```python
from build123d import *

# Parameters (mm, degrees)
F1_DEPTH = 3.175
F2_W     = 62.6118863001
F2_H     = 3.175
F3_DEPTH = 12.7
F4_SIZE  = 1.27
F5_W     = 15.875
F5_H     = 3.175
F6_DEPTH = 4.5143370517
F7_W     = 15.875
F7_H     = 3.175
F8_DEPTH = 4.3210691154


with BuildPart() as f1:
    # F0 (on Front) → F1 (new body)
    with BuildSketch(Plane.XZ):
        with BuildLine():
            ThreePointArc((-35.500738686, -3.175), (-34.8663710031, -1.6435009364), (-34.65, 0))
            Line((-34.65, 0), (-39.5, 0))
            ThreePointArc((-39.5, 0), (-41, -1.5), (-42.5, 0))
            Line((-42.5, 0), (-47.35, 0))
            ThreePointArc((-47.35, 0), (-47.1336289969, -1.6435009364), (-46.499261314, -3.175))
            Line((-46.499261314, -3.175), (-35.500738686, -3.175))
        make_face()
        with BuildLine():
            ThreePointArc((-40.777693324, 6.346107448), (-36.4319507778, 4.4108305685), (-34.65, 0))
            Line((-34.65, 0), (-6.35, 0))
            ThreePointArc((-6.35, 0), (-4.5680492222, 4.4108305685), (-0.222306676, 6.346107448))
            Line((-0.222306676, 6.346107448), (-40.777693324, 6.346107448))
        make_face()
        with BuildLine():
            Line((-39.5, 0), (-34.65, 0))
            ThreePointArc((-34.65, 0), (-36.4319507778, 4.4108305685), (-40.777693324, 6.346107448))
            ThreePointArc((-40.777693324, 6.346107448), (-45.4108305685, 4.5680492222), (-47.35, 0))
            Line((-47.35, 0), (-42.5, 0))
            ThreePointArc((-42.5, 0), (-41, 1.5), (-39.5, 0))
        make_face()
        with BuildLine():
            ThreePointArc((-46.499261314, -3.175), (-47.1336289969, -1.6435009364), (-47.35, 0))
            Line((-47.35, 0), (-47.35, -3.175))
            Line((-47.35, -3.175), (-46.499261314, -3.175))
        make_face()
        with BuildLine():
            ThreePointArc((-0.222306676, 6.346107448), (-4.5680492222, 4.4108305685), (-6.35, 0))
            Line((-6.35, 0), (-1.5, 0))
            ThreePointArc((-1.5, 0), (0, 1.5), (1.5, 0))
            Line((1.5, 0), (6.35, 0))
            ThreePointArc((6.35, 0), (4.4108305685, 4.5680492222), (-0.222306676, 6.346107448))
        make_face()
        with BuildLine():
            Line((-1.5, 0), (-6.35, 0))
            ThreePointArc((-6.35, 0), (-6.1336289969, -1.6435009364), (-5.499261314, -3.175))
            Line((-5.499261314, -3.175), (5.499261314, -3.175))
            ThreePointArc((5.499261314, -3.175), (6.1336289969, -1.6435009364), (6.35, 0))
            Line((6.35, 0), (1.5, 0))
            ThreePointArc((1.5, 0), (0, -1.5), (-1.5, 0))
        make_face()
        with BuildLine():
            Line((-51.6710691154, -6.35), (-41, -6.35))
            ThreePointArc((-41, -6.35), (-44.175, -5.499261314), (-46.499261314, -3.175))
            Line((-46.499261314, -3.175), (-47.35, -3.175))
            Line((-47.35, -3.175), (-51.6710691154, -3.175))
            Line((-51.6710691154, -3.175), (-51.6710691154, -6.35))
        make_face()
        with BuildLine():
            Line((-5.499261314, -3.175), (-35.500738686, -3.175))
            ThreePointArc((-35.500738686, -3.175), (-37.825, -5.499261314), (-41, -6.35))
            Line((-41, -6.35), (3.51e-08, -6.35))
            ThreePointArc((3.51e-08, -6.35), (-3.1749999848, -5.4992613228), (-5.499261314, -3.175))
        make_face()
        with BuildLine():
            ThreePointArc((5.499261314, -3.175), (3.1750000152, -5.4992613052), (3.51e-08, -6.35))
            Line((3.51e-08, -6.35), (10.9408171847, -6.35))
            Line((10.9408171847, -6.35), (10.9408171847, -3.175))
            Line((10.9408171847, -3.175), (6.4264801331, -3.175))
            Line((6.4264801331, -3.175), (5.499261314, -3.175))
        make_face()
        with BuildLine():
            Line((-51.6710691154, -6.35), (-41, -6.35))
            ThreePointArc((-41, -6.35), (-44.175, -5.499261314), (-46.499261314, -3.175))
            Line((-46.499261314, -3.175), (-47.35, -3.175))
            Line((-47.35, -3.175), (-51.6710691154, -3.175))
            Line((-51.6710691154, -3.175), (-51.6710691154, -6.35))
        make_face()
        with BuildLine():
            ThreePointArc((-41, -6.35), (-37.825, -5.499261314), (-35.500738686, -3.175))
            Line((-35.500738686, -3.175), (-46.499261314, -3.175))
            ThreePointArc((-46.499261314, -3.175), (-44.175, -5.499261314), (-41, -6.35))
        make_face()
        with BuildLine():
            Line((-6.35, 0), (-34.65, 0))
            ThreePointArc((-34.65, 0), (-34.8663710031, -1.6435009364), (-35.500738686, -3.175))
            Line((-35.500738686, -3.175), (-5.499261314, -3.175))
            ThreePointArc((-5.499261314, -3.175), (-6.1336289969, -1.6435009364), (-6.35, 0))
        make_face()
        with BuildLine():
            Line((5.499261314, -3.175), (-5.499261314, -3.175))
            ThreePointArc((-5.499261314, -3.175), (-3.1749999848, -5.4992613228), (3.51e-08, -6.35))
            ThreePointArc((3.51e-08, -6.35), (3.1750000152, -5.4992613052), (5.499261314, -3.175))
        make_face()
        with BuildLine():
            ThreePointArc((5.499261314, -3.175), (3.1750000152, -5.4992613052), (3.51e-08, -6.35))
            Line((3.51e-08, -6.35), (10.9408171847, -6.35))
            Line((10.9408171847, -6.35), (10.9408171847, -3.175))
            Line((10.9408171847, -3.175), (6.4264801331, -3.175))
            Line((6.4264801331, -3.175), (5.499261314, -3.175))
        make_face()
        with BuildLine():
            Line((6.4264801331, 0), (6.35, 0))
            ThreePointArc((6.35, 0), (6.1336289969, -1.6435009364), (5.499261314, -3.175))
            Line((5.499261314, -3.175), (6.4264801331, -3.175))
            Line((6.4264801331, -3.175), (6.4264801331, 0))
        make_face()
    extrude(amount=F1_DEPTH)

    # F2 (on face) → F3 (join)
    with BuildSketch(Plane.XZ.offset(3.175)):
        with Locations((-20.3651259653, -4.7625)):
            Rectangle(F2_W, F2_H)
    extrude(amount=F3_DEPTH)

    # F4
    f4_edges = [f1.edges().sort_by_distance(p)[0] for p in [
        (-39.5, 0, 0),
    ]]
    chamfer(f4_edges, length=F4_SIZE)

    # F5 (on face) → F6 (cut, through all)
    with BuildSketch(Plane.YZ.offset(10.9408171847)):
        with Locations((-7.9375, -4.7625)):
            Rectangle(F5_W, F5_H)
    extrude(amount=-F6_DEPTH, mode=Mode.SUBTRACT)

    # F7 (on face) → F8 (cut, through all)
    with BuildSketch(Plane(origin=(-51.6710691154, 0, 0), x_dir=(0, -1, 0), z_dir=(-1, 0, 0))):
        with Locations((7.9375, -4.7625)):
            Rectangle(F7_W, F7_H)
    extrude(amount=-F8_DEPTH, mode=Mode.SUBTRACT)


solid = f1.part
```
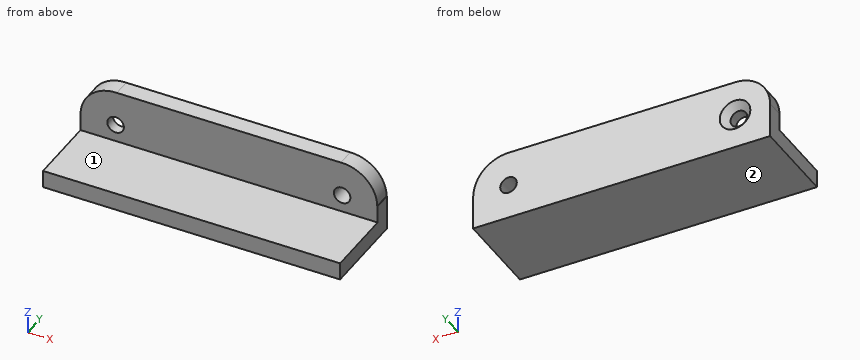
Source: CAD feature listing. Evaluate the final solid. Frame: model axes, mm. Face numbers are marked on the shaded views. A direction names the side the tool comes from. Coordinates: 2 decimals unless noted, no trailing zeros. Loops run counter-clockwise (first coordinate to the right, second up) from the corner with the lowest first, then second, coordinate; pieces in that order, holes last. Notation, with made-up numbers: M 18,61.25 L 27,61.25 A10 cw 27,77.25 Z; hole C 89.5,72 d1. An arc over 180 degrees is marked long. Use a Markdown table: item, result. Add a question column.
Q1. Section query C-C, the plane z = -0.5. State how many separate pieces and enclosed holes the cut face has, and give its area (3 significant figures).
Q2. Section query D-D, the plane y = -4.5. Return loops of the section in (x, z) (3 decimals).
Q3. Section query A-A, the plane y = -2. Return loops of the section in (x, z), and give its area (3 significant figures).
Q4. Material intervals for L1, parallel to Z at x = 0, y = -2.5; L2, parallel to X at y = -2.5, z = -0.25; L3, parallel to Z at x = -24.5, y = -13.5 (3 decimals), sorted ascending.
Q5. Access query for the marked faces 1 and 2. Directions: +Z, -Z, +X, -X, +Y, -Y. A direction counts if a zero-diameter tool reaches every point of the face in a straight line with its end or side. Return the directions, or none.
Q6. First-contact query: pin 1 (8 mm diameter, centred on x = -6.5, y = -12.5, fed in from +Z) (3 decimals); pin 2 (1.6 mm diameter, centred on x = -25.5, y = -1.5, fed in from +Z); pin 3 (2.5 mm diameter, centred on x = -41, z = 0, fed in from -Y); pin 4 (7.5 mm diameter, centred on x = -14, z = 1, fed in from -Y) (3 decimals). Flat tips, straight axial feed; report the tip coordinate or a pass-through.
Q7. Section query B-B, the plane x = -7. Return loops of the section in (y, z) (3 decimals), and give its area (3 significant figures).
Result:
| question | item | result |
|---|---|---|
| 1 | separate pieces | 3 |
| 1 | enclosed holes | 0 |
| 1 | area | 151 mm2 |
| 2 | outline | M -47.35,-6.35 L 6.426,-6.35 L 6.426,-3.175 L -47.35,-3.175 Z |
| 3 | outline | M -47.35,-6.35 L 6.43,-6.35 L 6.43,0 L 6.35,0 A6.35 ccw -0.22,6.35 L -40.78,6.35 A6.35 ccw -47.35,0 Z; hole C -41,0 d3; hole C 0,0 d3 |
| 3 | area | 651 mm2 |
| 4 | L1 | z = -6.35 to -1.5, 1.5 to 6.35 |
| 4 | L2 | x = -47.35 to -42.48, -39.52 to -1.48, 1.48 to 6.43 |
| 4 | L3 | z = -6.35 to -3.175 |
| 5 | face 1 | +Z, +X, -X, -Y |
| 5 | face 2 | -Z, +X, -X, +Y, -Y |
| 6 | pin 1 | stops at z = -3.175 |
| 6 | pin 2 | stops at z = 6.35 |
| 6 | pin 3 | passes through |
| 6 | pin 4 | stops at y = -3.175 |
| 7 | outline | M -15.875,-6.35 L 0,-6.35 L 0,6.346 L -3.175,6.346 L -3.175,-3.175 L -15.875,-3.175 Z |
| 7 | area | 80.6 mm2 |
